Autodesk Inventor part; units mm, degrees
ref_plane "YZ Plane" through (0, 0, 0) normal (1, 0, 0) x (0, 1, 0)
ref_plane "XZ Plane" through (0, 0, 0) normal (0, 1, 0) x (-1, 0, 0)
ref_plane "XY Plane" through (0, 0, 0) normal (0, 0, 1) x (1, 0, 0)
sketch "Base" plane through (0, 0, 0) normal (0, 0, 1) x (1, 0, 0)
  circle A0 centre (0, 0) radius 7.75
  line L0 (0, 0) -> (-20, 0) construction
  circle A1 centre (-20, 0) radius 7.75
  circle A2 centre (0, 0) radius 3
  circle A3 centre (-20, 0) radius 3
  line L1 (-20, 7.75) -> (0, 7.75)
  line L2 (-20, -7.75) -> (0, -7.75)
  dimension "d0" = 15.5
  dimension "d1" = 20
  dimension "d3" = 6
extrude "BaseFeature" add sketch "Base" along normal blind 3
properties part number "FaceTubeConnector"
Model file for the job. Use its own axes, mm. Coordinates: 2 decimals unless noted, no trailing zeros. Write each loop counter-clockwise with the first axis right and the second up, starting at its lowest first coordinate (ties: lowest second). Pieces come first, ordered by that corner, then holes. Notation, with made-up numbers: (-23, 85.5) - (0, 85.5) arc R17 ccw to (0, 96.5) - close; hole circle Ø1 at (-35.75, 12). An arc over 180 degrees is marked (long way). One line per item, written item: value. Start each with the question number.
1. Slice it at C-C (z = 0.8). Write the cut outline in (x, y), plus the area to 3 significant figures.
2. Slice it at D-D (x = 2). Write the cut outline in (y, z).
3. Slice it at A-A (y = 0). Write the cut outline in (x, z).
4. Mould opens along X. For faces 1 (the flat face through (-10, -7.75, 1)), 2 (the cylindrical face through (7.75, 0.17, 1.48)), 3 (the cylindrical face through (-23, 0, 1)) say: released by +X, released by -X, zero draft, split by the parting line, or undercut.
5. Probe line 1 (Y direction, x = 0, z = 1.5); line 2 (X direction, y = 1.5, z = 1.45). List the from-to ranges inside material, lowest first. Write a range as from..to.
6. Flat gauge pin, fed straight in: pin 1 (1.5 mm diameter, centred on y = -2.5, z = 1, fed in from +X). Where does the tip first touch, or does it go through?
7. Slice it at B-B (x = -17.5). Write the cut outline in (y, z).
Answers below:
1. outline: (-20, -7.75) - (0, -7.75) arc R7.75 ccw to (0, 7.75) - (-20, 7.75) arc R7.75 ccw to start; hole circle Ø6 at (-20, 0); hole circle Ø6 at (0, 0)
1. area: 442 mm^2
2. outline: (-7.49, 0) - (-2.24, 0) - (-2.24, 3) - (-7.49, 3) - close; (2.24, 0) - (7.49, 0) - (7.49, 3) - (2.24, 3) - close
3. outline: (-27.75, 0) - (-23, 0) - (-23, 3) - (-27.75, 3) - close; (-17, 0) - (-3, 0) - (-3, 3) - (-17, 3) - close; (3, 0) - (7.75, 0) - (7.75, 3) - (3, 3) - close
4. face 1: zero draft
4. face 2: released by +X
4. face 3: undercut
5. line 1: y = -7.75..-3, 3..7.75
5. line 2: x = -27.6..-22.6, -17.4..-2.6, 2.6..7.6
6. pin 1: stops at x = 7.55
7. outline: (-7.75, 0) - (-1.66, 0) - (-1.66, 3) - (-7.75, 3) - close; (1.66, 0) - (7.75, 0) - (7.75, 3) - (1.66, 3) - close
